Autodesk Inventor part; units mm, degrees
ref_plane "YZ Plane" through (0, 0, 0) normal (1, 0, 0) x (0, 1, 0)
ref_plane "XZ Plane" through (0, 0, 0) normal (0, 1, 0) x (-1, 0, 0)
ref_plane "XY Plane" through (0, 0, 0) normal (0, 0, 1) x (1, 0, 0)
sketch "Sketch1" plane through (0, 0, 0) normal (1, 0, 0) x (0, 1, 0)
  line L0 (2, 0) -> (18, 0)
  line L1 (20, -2) -> (20, -18)
  line L2 (18, -20) -> (2, -20)
  line L3 (0, -18) -> (0, -2)
  line L4 (18, -18) -> (18, -2)
  line L5 (18, -2) -> (2, -2)
  line L6 (2, -2) -> (2, -18)
  line L7 (2, -18) -> (18, -18)
  arc A0 (20, -2) -> (18, 0) centre (18, -2) ccw
  arc A1 (18, -20) -> (20, -18) centre (18, -18) ccw
  arc A2 (0, -18) -> (2, -20) centre (2, -18) ccw
  arc A3 (2, 0) -> (0, -2) centre (2, -2) ccw
  point P0 (0, 0)
  point P1 (20, -20)
  point P2 (20, 0)
  point P3 (0, -20)
  dimension "d0" = 20
  dimension "d1" = 20
  dimension "d2" = 2
  dimension "d5" = 2
extrude "Extrusion1" add sketch "Sketch1" along normal blind 319
sketch "Sketch2" plane through (0, 0, -18) normal (0, -1, 0) x (1, 0, 0)
  line L0 (0, 16) -> (0, 0)
  line L1 (0, 0) -> (319, 0)
  point P0 (0, 18)
  point P1 (16, 8)
  dimension "d6" = 16
  dimension "d7" = 8
hole "Hole1" at (16, 0, -10) direction (0, 1, 0) diameter 2.45 depth 2
sketch "Sketch4" plane through (0, 2, -20) normal (0, 0, -1) x (-1, 0, 0)
  line L0 (0, 0) -> (0, 16)
  line L1 (0, 16) -> (-319, 16)
  line L2 (0, 0) -> (-16, 0)
  line L3 (-16, 0) -> (-16, 16)
  line L4 (-16, 16) -> (0, 16)
  line L5 (0, 16) -> (0, 0)
  point P0 (0, -2)
extrude "Extrusion3" cut sketch "Sketch4" against normal up to surface (2 mm away)
properties part number "rockerpivotarm"
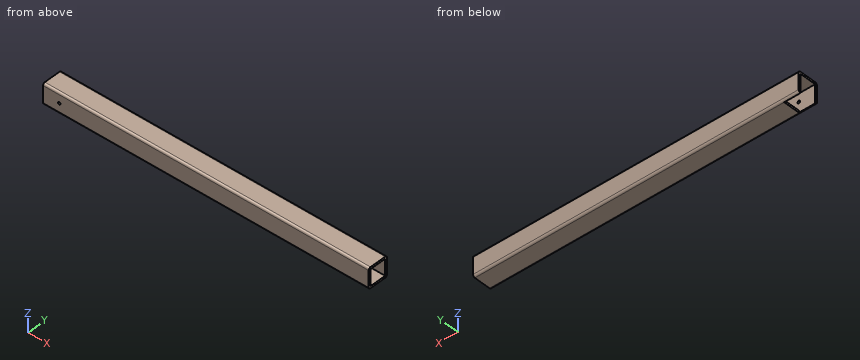
Input: part model. Units: mm. Frame: model coordinates. Coordinates: 2 decimals unless noted, no trailing zeros. Loops run counter-clockwise (first coordinate to the right, second up) from the corner with the lowest first, then second, coordinate; pieces in that order, holes last.
(1) Material intervals for probe 1 along Z at (x, y) = (159.5, 17.5); probe 2 along X at (y, z) = (0.6, -10) (3 decimals); probe 3 along Y at (x, z) = (132, -16.5), sorted ascending.
(2) Section B-B on x = 100.5. Return the cut outline in (y, z).
(3) First-contact query: pin 1 Ø1.6 at (y, z) = (13, -19.5) entering from -X. Flat tip, straight axial feed; report the tip coordinate or a pass-through.
(4) Section A-A on z = -14.5. Return the cut outline in (x, y).
Data:
1. probe 1: z = -20 to -18, -2 to 0
1. probe 2: x = 0 to 14.775, 17.225 to 319
1. probe 3: y = 0 to 2, 18 to 20
2. outline: (0, -18) arc R2 ccw to (2, -20) - (18, -20) arc R2 ccw to (20, -18) - (20, -2) arc R2 ccw to (18, 0) - (2, 0) arc R2 ccw to (0, -2) - close; hole (2, -18) - (18, -18) - (18, -2) - (2, -2) - close
3. pin 1: stops at x = 16
4. outline: (0, 0) - (319, 0) - (319, 2) - (0, 2) - close; (0, 18) - (319, 18) - (319, 20) - (0, 20) - close
